from build123d import *

# Parameters (mm, degrees)
F0_R     = 31
F1_DEPTH = 5


with BuildPart() as f1:
    # F0 (on Top) → F1 (new body)
    with BuildSketch(Plane.XY):
        Circle(F0_R)
        with BuildLine():
            ThreePointArc((-28.7080992435, 1.5), (-27.1015041114, 3.4034806404), (-24.68, 3.9871794542))
            ThreePointArc((-24.68, 3.9871794542), (-23.1340148639, 9.4772019223), (-20.3839350968, 14.4739486654))
            ThreePointArc((-20.3839350968, 14.4739486654), (-21.7843066075, 16.7218663809), (-21.4732899684, 19.3519696248))
            Line((-21.4732899684, 19.3519696248), (-21.9870643658, 19.8657440223))
            Line((-21.9870643658, 19.8657440223), (-19.8657440223, 21.9870643658))
            Line((-19.8657440223, 21.9870643658), (-19.2357510946, 21.3570714382))
            ThreePointArc((-19.2357510946, 21.3570714382), (-16.8275788969, 21.4526090468), (-14.8016328487, 20.1472495644))
            ThreePointArc((-14.8016328487, 20.1472495644), (-8.7324141696, 23.4253056068), (-1.9983993595, 24.92))
            ThreePointArc((-1.9983993595, 24.92), (-0.0400080056, 26.9995997998), (2, 25))
            ThreePointArc((2, 25), (1.9995997998, 24.9599919944), (1.9983993595, 24.92))
            ThreePointArc((1.9983993595, 24.92), (8.396839067, 23.5476770337), (14.2199501873, 20.5619312485))
            ThreePointArc((14.2199501873, 20.5619312485), (16.578332036, 21.8337211242), (19.2103126472, 21.3316329908))
            Line((19.2103126472, 21.3316329908), (19.8657440223, 21.9870643658))
            Line((19.8657440223, 21.9870643658), (21.9870643658, 19.8657440223))
            Line((21.9870643658, 19.8657440223), (21.048652157, 18.9273318134))
            ThreePointArc((21.048652157, 18.9273318134), (21.1530642912, 18.408521084), (21.1880725996, 17.8804672182))
            ThreePointArc((21.1880725996, 17.8804672182), (20.8749504136, 16.3290382046), (19.9846066074, 15.020502613))
            ThreePointArc((19.9846066074, 15.020502613), (22.9196691944, 9.9844260737), (24.608757715, 4.4055696256))
            ThreePointArc((24.608757715, 4.4055696256), (27.0107687706, 3.5932566366), (28.4417775606, 1.5))
            Line((28.4417775606, 1.5), (29.5944046229, 1.5))
            Line((29.5944046229, 1.5), (29.5944046229, -1.5))
            Line((29.5944046229, -1.5), (28.1113217756, -1.5))
            ThreePointArc((28.1113217756, -1.5), (26.7035545193, -2.9931524386), (24.7406441339, -3.5917304797))
            ThreePointArc((24.7406441339, -3.5917304797), (23.2131665144, -9.2816431936), (20.3965858209, -14.4561158978))
            ThreePointArc((20.3965858209, -14.4561158978), (21.1955475808, -15.7195454325), (21.4748718411, -17.1880725996))
            ThreePointArc((21.4748718411, -17.1880725996), (21.3717482185, -18.0904885234), (21.0676945913, -18.9463742477))
            Line((21.0676945913, -18.9463742477), (21.9870643658, -19.8657440223))
            Line((21.9870643658, -19.8657440223), (19.8657440223, -21.9870643658))
            Line((19.8657440223, -21.9870643658), (18.8301557175, -20.9514760611))
            ThreePointArc((18.8301557175, -20.9514760611), (16.7005194557, -21.1124041838), (14.7916340459, -20.1545915923))
            ThreePointArc((14.7916340459, -20.1545915923), (9.6637784532, -23.0566993737), (3.9991249765, -24.6780671736))
            ThreePointArc((3.9991249765, -24.6780671736), (3.2930577298, -26.865036867), (1.5, -28.3025038665))
            Line((1.5, -28.3025038665), (1.5, -29.5944046229))
            Line((1.5, -29.5944046229), (-1.5, -29.5944046229))
            Line((-1.5, -29.5944046229), (-1.5, -28.3025038665))
            ThreePointArc((-1.5, -28.3025038665), (-3.2930577298, -26.865036867), (-3.9991249765, -24.6780671736))
            ThreePointArc((-3.9991249765, -24.6780671736), (-9.606613518, -23.0805757449), (-14.691565202, -20.2276521602))
            ThreePointArc((-14.691565202, -20.2276521602), (-16.7333297142, -21.3812535524), (-19.0708139147, -21.1921342582))
            Line((-19.0708139147, -21.1921342582), (-19.8657440223, -21.9870643658))
            Line((-19.8657440223, -21.9870643658), (-21.9870643658, -19.8657440223))
            Line((-21.9870643658, -19.8657440223), (-21.2402040172, -19.1188836736))
            ThreePointArc((-21.2402040172, -19.1188836736), (-21.5159012518, -16.6899602951), (-20.326723356, -14.5541855701))
            ThreePointArc((-20.326723356, -14.5541855701), (-23.115291289, -9.522778409), (-24.68, -3.9871794542))
            ThreePointArc((-24.68, -3.9871794542), (-27.1015041114, -3.4034806404), (-28.7080992435, -1.5))
            Line((-28.7080992435, -1.5), (-29.5944046229, -1.5))
            Line((-29.5944046229, -1.5), (-29.5944046229, 1.5))
            Line((-29.5944046229, 1.5), (-28.7080992435, 1.5))
        make_face(mode=Mode.SUBTRACT)
        with BuildLine():
            ThreePointArc((-24.68, 3.9871794542), (-22.6329530448, 3.2244516916), (-21.2919007565, 1.5))
            Line((-21.2919007565, 1.5), (-19.5944046229, 1.5))
            Line((-19.5944046229, 1.5), (-19.5944046229, -1.5))
            Line((-19.5944046229, -1.5), (-21.2919007565, -1.5))
            ThreePointArc((-21.2919007565, -1.5), (-22.6329530448, -3.2244516916), (-24.68, -3.9871794542))
            ThreePointArc((-24.68, -3.9871794542), (-23.115291289, -9.522778409), (-20.326723356, -14.5541855701))
            ThreePointArc((-20.326723356, -14.5541855701), (-18.2480519875, -13.5287621662), (-15.9496561442, -13.8283358006))
            Line((-15.9496561442, -13.8283358006), (-14.915996554, -12.7946762104))
            Line((-14.915996554, -12.7946762104), (-12.7946762104, -14.915996554))
            Line((-12.7946762104, -14.915996554), (-13.8764055595, -15.9977259031))
            ThreePointArc((-13.8764055595, -15.9977259031), (-13.664988194, -16.7228910131), (-13.5936679767, -17.4748718411))
            ThreePointArc((-13.5936679767, -17.4748718411), (-13.8782668477, -18.95669317), (-14.691565202, -20.2276521602))
            ThreePointArc((-14.691565202, -20.2276521602), (-9.606613518, -23.0805757449), (-3.9991249765, -24.6780671736))
            ThreePointArc((-3.9991249765, -24.6780671736), (-3.3398290754, -22.3931454952), (-1.5, -20.8863053794))
            Line((-1.5, -20.8863053794), (-1.5, -19.5944046229))
            Line((-1.5, -19.5944046229), (1.5, -19.5944046229))
            Line((1.5, -19.5944046229), (1.5, -20.8863053794))
            ThreePointArc((1.5, -20.8863053794), (3.3166247904, -22.3583366454), (4, -24.5944046229))
            ThreePointArc((4, -24.5944046229), (3.9997812381, -24.6362381861), (3.9991249765, -24.6780671736))
            ThreePointArc((3.9991249765, -24.6780671736), (9.6637784532, -23.0566993737), (14.7916340459, -20.1545915923))
            ThreePointArc((14.7916340459, -20.1545915923), (13.5942416238, -18.1579742011), (13.7114683796, -15.8327887231))
            Line((13.7114683796, -15.8327887231), (12.7946762104, -14.915996554))
            Line((12.7946762104, -14.915996554), (14.915996554, -12.7946762104))
            Line((14.915996554, -12.7946762104), (15.716570193, -13.5952498494))
            ThreePointArc((15.716570193, -13.5952498494), (18.1985117044, -13.2540739534), (20.3965858209, -14.4561158978))
            ThreePointArc((20.3965858209, -14.4561158978), (23.2131665144, -9.2816431936), (24.7406441339, -3.5917304797))
            ThreePointArc((24.7406441339, -3.5917304797), (22.6109225733, -3.0679905163), (21.0774874702, -1.5))
            Line((21.0774874702, -1.5), (19.5944046229, -1.5))
            Line((19.5944046229, -1.5), (19.5944046229, 1.5))
            Line((19.5944046229, 1.5), (20.7470316853, 1.5))
            ThreePointArc((20.7470316853, 1.5), (22.1894942303, 3.6019066891), (24.608757715, 4.4055696256))
            ThreePointArc((24.608757715, 4.4055696256), (22.9196691944, 9.9844260737), (19.9846066074, 15.020502613))
            ThreePointArc((19.9846066074, 15.020502613), (18.1958639143, 14.0095039446), (16.1412080043, 14.0198876608))
            Line((16.1412080043, 14.0198876608), (14.915996554, 12.7946762104))
            Line((14.915996554, 12.7946762104), (12.7946762104, 14.915996554))
            Line((12.7946762104, 14.915996554), (13.736906827, 15.8582271706))
            ThreePointArc((13.736906827, 15.8582271706), (13.2089994395, 18.2890951502), (14.2199501873, 20.5619312485))
            ThreePointArc((14.2199501873, 20.5619312485), (8.396839067, 23.5476770337), (1.9983993595, 24.92))
            ThreePointArc((1.9983993595, 24.92), (0, 23), (-1.9983993595, 24.92))
            ThreePointArc((-1.9983993595, 24.92), (-8.7324141696, 23.4253056068), (-14.8016328487, 20.1472495644))
            ThreePointArc((-14.8016328487, 20.1472495644), (-14.1177994493, 18.9509930155), (-13.8804672182, 17.5936679767))
            ThreePointArc((-13.8804672182, 17.5936679767), (-13.9400602693, 16.9057776679), (-14.1170637567, 16.2383841002))
            Line((-14.1170637567, 16.2383841002), (-12.7946762104, 14.915996554))
            Line((-12.7946762104, 14.915996554), (-14.915996554, 12.7946762104))
            Line((-14.915996554, 12.7946762104), (-16.12216557, 14.0008452265))
            ThreePointArc((-16.12216557, 14.0008452265), (-18.3218003053, 13.618089389), (-20.3839350968, 14.4739486654))
            ThreePointArc((-20.3839350968, 14.4739486654), (-23.1340148639, 9.4772019223), (-24.68, 3.9871794542))
        make_face()
        with BuildLine():
            ThreePointArc((1.5, 3.9764934301), (3.4955328635, 2.4173849507), (4.25, 0))
            ThreePointArc((4.25, 0), (3.4955328635, -2.4173849507), (1.5, -3.9764934301))
            Line((1.5, -3.9764934301), (1.5, -4.75))
            Line((1.5, -4.75), (-1.5, -4.75))
            Line((-1.5, -4.75), (-1.5, -3.9764934301))
            ThreePointArc((-1.5, -3.9764934301), (-4.25, 0), (-1.5, 3.9764934301))
            Line((-1.5, 3.9764934301), (-1.5, 4.75))
            Line((-1.5, 4.75), (1.5, 4.75))
            Line((1.5, 4.75), (1.5, 3.9764934301))
        make_face(mode=Mode.SUBTRACT)
    extrude(amount=F1_DEPTH)


solid = f1.part
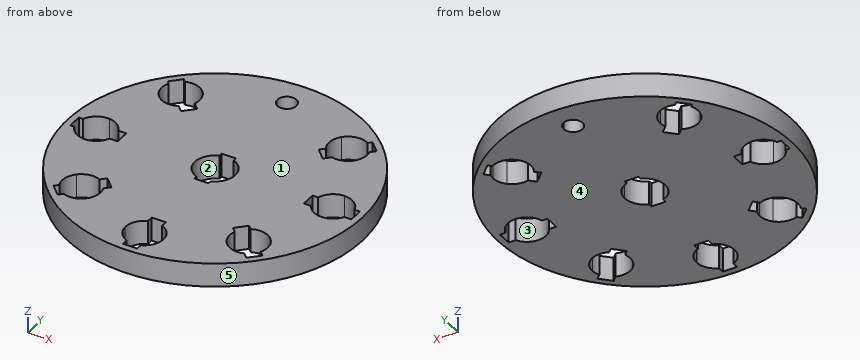
The listing builds one solid part. Answer for the finished solid, in the listing's coordinates (mm). Face numbers are marked on the shaded views. A direction names the side the tool comes from. Coordinates: 2 decimals unless noted, no trailing zeros. Write each loop counter-clockwise with the first axis right and the second up, starting at its lowest first coordinate (ties: lowest second). Pieces come first, ordered by that corner, then holes. Notation, with made-up numbers: (12.5, 23.5) - (29.5, 23.5) arc R9 ccw to (29.5, 32.5) - close; hole circle Ø11 at (46, 34). An arc over 180 degrees is marked (long way). Return JSON: item names as keys, results as strings.
1. The part is cut by section C-C on y = 10.5. Determine the outline of the cut face in (x, z), then the cut area to 3 significant figures.
Final values:
{"outline": "(-29.17, 0) - (29.17, 0) - (29.17, 5) - (-29.17, 5) - close", "area": "292 mm^2"}
2. Which of the six approach directions +Z, -Z, +X, -X, +Y, -Y give full straight-line access (tool end or side, diameter ignored) to the marked faces 1 and 2?
Final values:
{"face 1": "+Z, +X, -X, +Y, -Y", "face 2": "+Z, -Z"}
3. For a pull along X with two mould halves and no side action, classify the marked faces 3, 4 and 5 as +X half, -X half, draft (parallel to the pull), parting line (faces both ways), or undercut.
Final values:
{"face 3": "undercut", "face 4": "draft", "face 5": "parting line"}
4. The part is cut by section B-B on z = 3.15. Count the separate pieces of the cut face and the enclosed holes in it, then the cut area to 3 significant figures.
Final values:
{"separate pieces": "1", "enclosed holes": "9", "area": "2,550 mm^2"}
5. Each of these flat-tipped pins is pushed along its axis until it touches: pin 1 Ø3 at (x, z) = (-2, 3.5) entering from -Y; pin 2 Ø1 at (y, z) = (-21, 4) entering from +X; pin 3 Ø1.5 at (x, z) = (0, 3) entering from +Y. Where does it stop, or does it pass through?
Final values:
{"pin 1": "y = -31", "pin 2": "x = 23.25", "pin 3": "y = 31"}
6. Consider line 1 along Y through (x, z) = (-3.5, 1.2); line 2 along Y through (x, z) = (17, 4.45); line 3 along X through (y, z) = (-2, 1.55). Determine where each line is inside the solid, lowest interval first.
Final values:
{"line 1": "-30.8 to -26.53, -22.66 to -2.41, 2.41 to 30.8", "line 2": "-25.92 to -21.16, -13.22 to 13.88, 21.88 to 25.92", "line 3": "-30.94 to -28.46, -21.54 to -3.75, 3.75 to 21.4, 27.79 to 30.94"}
7. The part is cut by section D-D on y = -7.5. Determine the outline of the cut face in (x, z).
Final values:
{"outline": "(-30.08, 0) - (30.08, 0) - (30.08, 5) - (-30.08, 5) - close"}
8. The part is cut by section A-A on x = 0. Determine the outline of the cut face in (y, z).
Final values:
{"outline": "(-31, 0) - (-29.59, 0) - (-29.59, 5) - (-31, 5) - close; (-19.59, 0) - (-4.75, 0) - (-4.75, 5) - (-19.59, 5) - close; (4.75, 0) - (23, 0) - (23, 5) - (4.75, 5) - close; (27, 0) - (31, 0) - (31, 5) - (27, 5) - close"}
